Read the model definition and answer for the solid it produces. Units are mm, in the model's axes. A direction names the side the tool comes from. Give positions to 0.01 mm unless a question says otherwise; leave off trailing zeros. Order: outer loops, then holes, each group sorted by start corner. A loop starts at its lowest first (then second) coordinate and runs counter-clockwise, first axis right, second up.
Item 1: A cutting plane is placed at A-A (y = -3). Write down the section's boundary in (x, z).
Item 2: Which of the six approach directions +Z, -Z, +X, -X, +Y, -Y give full straight-line access (tool end or side, diameter ignored) to faces 1 (the face through (-13, -3, -19.296)), 2 (the face through (8.846, -4, 12)), 3 (the face through (-13, -3, 52.182))?
Item 3: A cutting plane is placed at C-C (z = -4). Write down the section's boundary in (x, y).
Item 4: The mould has two halves that part along Z. Classify faces 4 (the face through (-7.286, -3.131, 53.086)), 5 (the face through (-13, 0, 17)), 6 (the face through (-26.454, -3.131, 57.852)): +Z half, -Z half, draft (parallel to the pull), parting line (faces both ways), or undercut.
Item 5: A cutting plane is placed at B-B (z = 57.5). Write down the section's boundary in (x, y).
Item 6: A cutting plane is placed at D-D (x = -15). Write down the section's boundary in (y, z).
Item 7: Find the intervals of material crossed by line 1 along X through (y, z) = (-5.5, 33); line 2 along Z through (x, y) = (4, -4.5); line 3 along Z through (x, y) = (-17, -5.5), in increasing order.
Item 8: Given pin 1 Ø13 at (x, z) = (-10, 11.5) entering from -Y; pin 2 Ø3.5 at (x, y) = (-21.5, -3.5) entering from +Z, each flat-ended and moving along its own axis, determine where each tip first touches the part or whether it passes through.
from build123d import *

# Parameters (mm, degrees)
F1_DEPTH     = 6.35
F2_W         = 43.0978981023
F2_H         = 50.8
F3_DEPTH     = 4.318
F5_DEPTH     = 6.35
F7_DEPTH     = 6.351
F8_T1_DEPTH  = 6.35
F8_T3_DEPTH  = 6.35
F8_T5_DEPTH  = 6.35
F8_T7_DEPTH  = 13.7467402192
F8_T9_DEPTH  = 14.3479140779
F8_T11_DEPTH = 13.97
F8_T13_DEPTH = 13.97
F8_T15_DEPTH = 13.724225926


# Not quite as in the source:
# - a fillet or chamfer that OpenCascade refuses, or shapes differently, is made with other operations: its cross-section is extruded or revolved along the edge and cut away or added


with BuildPart() as f1:
    # F0 (on Front) → F1 (new body)
    with BuildSketch(Plane.XZ):
        Polygon((-40.601760045, 44.2037712147), (-40.601760045, 20.0136204353), (-40.601760045, -19.2962287853), (-31.9894673416, -19.2962287853), (6.5923849878, -19.2962287853), (15.1961380572, -19.2962287853), (15.1961380572, 20.0136204353), (15.1961380572, 44.2037712147), align=None)
    extrude(amount=F1_DEPTH)

    # F2 (on face) → F3 (cut, through all)
    with BuildSketch(Plane.XZ.offset(6.35)):
        with Locations((-12.7028109939, 12.4537712147)):
            Rectangle(F2_W, F2_H)
    extrude(amount=-F3_DEPTH, mode=Mode.SUBTRACT)

    # F4 (on Front) → F5 (join, through all)
    with BuildSketch(Plane.XZ):
        Polygon((-12.7028109939, 72.2804571797), (-39.4616971228, 44.2037712147), (14.0383420512, 44.2037712147), align=None)
    extrude(amount=F5_DEPTH)

    # F6 (on Front) → F7 (cut, through all)
    with BuildSketch(Plane.XZ):
        Polygon((-5.3985980339, 52.1819666028), (-12.8735816106, 61.0412061214), (-20.9022667259, 52.1819666028), align=None)
    extrude(amount=F7_DEPTH, mode=Mode.SUBTRACT)

    # F8: fillet of radius 1.524 on 8 edges, made by hand

    # F8_s2 → F8_t1 (join)
    with BuildSketch(Plane.XZ):
        with BuildLine():
            ThreePointArc((-11.7497792539, 59.7092922586), (-12.8875838111, 60.2502701687), (-14.0438236179, 59.7499044838))
            Line((-14.0438236179, 59.7499044838), (-12.8735816106, 61.0412061214))
            Line((-12.8735816106, 61.0412061214), (-11.7497792539, 59.7092922586))
        make_face()
    extrude(amount=F8_T1_DEPTH)

    # F8_s4 → F8_t3 (join)
    with BuildSketch(Plane.XZ):
        with BuildLine():
            ThreePointArc((-7.5136965339, 54.688749932), (-7.2963881401, 53.0637772981), (-8.6784767396, 52.1819666028))
            Line((-8.6784767396, 52.1819666028), (-5.3985980339, 52.1819666028))
            Line((-5.3985980339, 52.1819666028), (-7.5136965339, 54.688749932))
        make_face()
    extrude(amount=F8_T3_DEPTH)

    # F8_s6 → F8_t5 (join)
    with BuildSketch(Plane.XZ):
        with BuildLine():
            ThreePointArc((-17.4644255473, 52.1819666028), (-18.8576647272, 53.0883416458), (-18.5936897056, 54.7293621572))
            Line((-18.5936897056, 54.7293621572), (-20.9022667259, 52.1819666028))
            Line((-20.9022667259, 52.1819666028), (-17.4644255473, 52.1819666028))
        make_face()
    extrude(amount=F8_T5_DEPTH)

    # F8_s8 → F8_t7 (cut)
    with BuildSketch(Plane.XZ.offset(-3.6983701096)):
        with BuildLine():
            ThreePointArc((14.0383420512, 44.2037712147), (14.8722778172, 43.6636997843), (15.1961380572, 42.7244231708))
            Line((15.1961380572, 42.7244231708), (15.1961380572, 44.2037712147))
            Line((15.1961380572, 44.2037712147), (14.0383420512, 44.2037712147))
        make_face()
    extrude(amount=F8_T7_DEPTH, mode=Mode.SUBTRACT)

    # F8_s10 → F8_t9 (cut)
    with BuildSketch(Plane.XZ.offset(-3.9989570389)):
        with BuildLine():
            ThreePointArc((-11.5996190182, 71.1221685073), (-12.7029244443, 71.5951040748), (-13.8063863853, 71.122533806))
            Line((-13.8063863853, 71.122533806), (-12.7028109939, 72.2804571797))
            Line((-12.7028109939, 72.2804571797), (-11.5996190182, 71.1221685073))
        make_face()
    extrude(amount=F8_T9_DEPTH, mode=Mode.SUBTRACT)

    # F8_s12 → F8_t11 (cut)
    with BuildSketch(Plane.XZ.offset(-3.81)):
        with BuildLine():
            ThreePointArc((15.1961380572, -17.7722287853), (14.7497687918, -18.8498595199), (13.6721380572, -19.2962287853))
            Line((13.6721380572, -19.2962287853), (15.1961380572, -19.2962287853))
            Line((15.1961380572, -19.2962287853), (15.1961380572, -17.7722287853))
        make_face()
    extrude(amount=F8_T11_DEPTH, mode=Mode.SUBTRACT)

    # F8_s14 → F8_t13 (cut)
    with BuildSketch(Plane.XZ.offset(-3.81)):
        with BuildLine():
            ThreePointArc((-39.077760045, -19.2962287853), (-40.1553907795, -18.8498595199), (-40.601760045, -17.7722287853))
            Line((-40.601760045, -17.7722287853), (-40.601760045, -19.2962287853))
            Line((-40.601760045, -19.2962287853), (-39.077760045, -19.2962287853))
        make_face()
    extrude(amount=F8_T13_DEPTH, mode=Mode.SUBTRACT)

    # F8_s16 → F8_t15 (cut)
    with BuildSketch(Plane.XZ.offset(-3.687112963)):
        with BuildLine():
            ThreePointArc((-40.601760045, 42.7289260295), (-40.2835162614, 43.6609817932), (-39.4616971228, 44.2037712147))
            Line((-39.4616971228, 44.2037712147), (-40.601760045, 44.2037712147))
            Line((-40.601760045, 44.2037712147), (-40.601760045, 42.7289260295))
        make_face()
    extrude(amount=F8_T15_DEPTH, mode=Mode.SUBTRACT)


solid = f1.part
Response values:
1. outline: (-40.6, -17.77) arc R1.52 ccw to (-39.08, -19.3) - (13.67, -19.3) arc R1.52 ccw to (15.2, -17.77) - (15.2, 42.72) arc R1.52 ccw to (14.04, 44.2) - (-11.6, 71.12) arc R1.52 ccw to (-13.81, 71.12) - (-39.46, 44.2) arc R1.52 ccw to (-40.6, 42.73) - close; hole (-34.25, -12.95) - (8.85, -12.95) - (8.85, 37.85) - (-34.25, 37.85) - close; hole (-18.59, 54.73) arc R1.52 ccw to (-17.46, 52.18) - (-8.68, 52.18) arc R1.52 ccw to (-7.51, 54.69) - (-11.75, 59.71) arc R1.52 ccw to (-14.04, 59.75) - close
2. face 1: -Z, +X, -X, +Y, -Y
2. face 2: -Y
2. face 3: +Y, -Y
3. outline: (-40.6, -6.35) - (-34.25, -6.35) - (-34.25, -2.03) - (8.85, -2.03) - (8.85, -6.35) - (15.2, -6.35) - (15.2, 0) - (-40.6, 0) - close
4. face 4: undercut
4. face 5: draft
4. face 6: +Z half
5. outline: (-26.79, -6.35) - (-16.08, -6.35) - (-16.08, 0) - (-26.79, 0) - close; (-9.89, -6.35) - (1.37, -6.35) - (1.37, 0) - (-9.89, 0) - close
6. outline: (-6.35, -19.3) - (0, -19.3) - (0, 52.18) - (-6.35, 52.18) - (-6.35, 37.85) - (-2.03, 37.85) - (-2.03, -12.95) - (-6.35, -12.95) - close; (-6.35, 58.69) - (0, 58.69) - (0, 69.87) - (-6.35, 69.87) - close
7. line 1: x = -40.6 to -34.25, 8.85 to 15.2
7. line 2: z = -19.3 to -12.95, 37.85 to 54.74
7. line 3: z = -19.3 to -12.95, 37.85 to 52.18, 56.49 to 67.77
8. pin 1: stops at y = -2.03
8. pin 2: stops at z = 64.89
